Verification items for the finished model (mm, model axes). A direction names the side the tool comes from. Round coordinates to 2 decimals unless told otherwise and drop trailing zeros. Loops run counter-clockwise (first coordinate to the right, second up) from the corner with the lowest first, then second, coordinate; pieces in that order, holes last. Notation, with made-up numbers: M -38.5,53.25 L -0.5,53.25 A22 cw -0.5,65.25 Z; hole C -8.5,51 d3. An arc over 180 degrees is marked long. One line per item, written item: value.
from build123d import *

# Parameters (mm, degrees)
MODEL_R                 = 2
MODEL_R_2               = 1.5
MODEL_R_3               = 4.5
SALIENTE_EXTRUIR1_DEPTH = 3


with BuildPart() as part:
    # Model → Saliente-Extruir1 (new body)
    with BuildSketch(Plane.XY):
        with BuildLine():
            Line((53.427599038, 287.872856798), (56.220729127, 292.710700024))
            ThreePointArc((56.220729127, 292.710700024), (50.061313425, 295.08905988), (43.537923027, 296.109047676))
            Line((43.537923027, 296.109047676), (43.537923027, 290.522787498))
            Line((43.537923027, 290.522787498), (40.537923027, 290.522787498))
            Line((40.537923027, 290.522787498), (40.537923027, 296.109047676))
            ThreePointArc((40.537923027, 296.109047676), (34.014532629, 295.08905988), (27.855116927, 292.710700024))
            Line((27.855116927, 292.710700024), (30.648247016, 287.872856798))
            Line((30.648247016, 287.872856798), (28.050170805, 286.372856798))
            Line((28.050170805, 286.372856798), (25.257040716, 291.210700024))
            ThreePointArc((25.257040716, 291.210700024), (20.11761281, 287.065669482), (15.972582269, 281.926241576))
            Line((15.972582269, 281.926241576), (20.810425495, 279.133111488))
            Line((20.810425495, 279.133111488), (19.310425495, 276.535035276))
            Line((19.310425495, 276.535035276), (14.472582269, 279.328165365))
            ThreePointArc((14.472582269, 279.328165365), (12.094222412, 273.168749664), (11.074234616, 266.645359265))
            Line((11.074234616, 266.645359265), (16.660494794, 266.645359265))
            Line((16.660494794, 266.645359265), (16.660494794, 263.645359265))
            Line((16.660494794, 263.645359265), (11.074234616, 263.645359265))
            ThreePointArc((11.074234616, 263.645359265), (12.094222412, 257.121968867), (14.472582269, 250.962553166))
            Line((14.472582269, 250.962553166), (19.310425495, 253.755683255))
            Line((19.310425495, 253.755683255), (20.810425495, 251.157607043))
            Line((20.810425495, 251.157607043), (15.972582269, 248.364476954))
            ThreePointArc((15.972582269, 248.364476954), (20.11761281, 243.225049049), (25.257040716, 239.080018507))
            Line((25.257040716, 239.080018507), (28.050170805, 243.917861733))
            Line((28.050170805, 243.917861733), (30.648247016, 242.417861733))
            Line((30.648247016, 242.417861733), (27.855116927, 237.580018507))
            ThreePointArc((27.855116927, 237.580018507), (34.014532629, 235.20165865), (40.537923027, 234.181670855))
            Line((40.537923027, 234.181670855), (40.537923027, 239.767931032))
            Line((40.537923027, 239.767931032), (43.537923027, 239.767931032))
            Line((43.537923027, 239.767931032), (43.537923027, 234.181670855))
            ThreePointArc((43.537923027, 234.181670855), (50.061313425, 235.20165865), (56.220729127, 237.580018507))
            Line((56.220729127, 237.580018507), (53.427599038, 242.417861733))
            Line((53.427599038, 242.417861733), (56.025675249, 243.917861733))
            Line((56.025675249, 243.917861733), (58.818805338, 239.080018507))
            ThreePointArc((58.818805338, 239.080018507), (63.958233244, 243.225049049), (68.103263786, 248.364476954))
            Line((68.103263786, 248.364476954), (63.26542056, 251.157607043))
            Line((63.26542056, 251.157607043), (64.76542056, 253.755683255))
            Line((64.76542056, 253.755683255), (69.603263786, 250.962553166))
            ThreePointArc((69.603263786, 250.962553166), (71.981623642, 257.121968867), (73.001611438, 263.645359265))
            Line((73.001611438, 263.645359265), (67.41535126, 263.645359265))
            Line((67.41535126, 263.645359265), (67.41535126, 266.645359265))
            Line((67.41535126, 266.645359265), (73.001611438, 266.645359265))
            ThreePointArc((73.001611438, 266.645359265), (71.981623642, 273.168749664), (69.603263786, 279.328165365))
            Line((69.603263786, 279.328165365), (64.76542056, 276.535035276))
            Line((64.76542056, 276.535035276), (63.26542056, 279.133111488))
            Line((63.26542056, 279.133111488), (68.103263786, 281.926241576))
            ThreePointArc((68.103263786, 281.926241576), (63.958233244, 287.065669482), (58.818805338, 291.210700024))
            Line((58.818805338, 291.210700024), (56.025675249, 286.372856798))
            Line((56.025675249, 286.372856798), (53.427599038, 287.872856798))
        make_face()
        with Locations((42.037923027, 265.145359265)):
            Circle(MODEL_R, mode=Mode.SUBTRACT)
        with Locations((39.708551621, 273.838691702)):
            Circle(MODEL_R_2, mode=Mode.SUBTRACT)
        with Locations((44.367294433, 256.452026829)):
            Circle(MODEL_R_2, mode=Mode.SUBTRACT)
        with Locations((42.037923027, 281.644073382)):
            Circle(MODEL_R_3, mode=Mode.SUBTRACT)
        with Locations((27.749617473, 273.394716324)):
            Circle(MODEL_R_3, mode=Mode.SUBTRACT)
        with Locations((27.749617473, 256.896002207)):
            Circle(MODEL_R_3, mode=Mode.SUBTRACT)
        with Locations((42.037923027, 248.646645149)):
            Circle(MODEL_R_3, mode=Mode.SUBTRACT)
        with Locations((56.326228582, 256.896002207)):
            Circle(MODEL_R_3, mode=Mode.SUBTRACT)
        with Locations((56.326228582, 273.394716324)):
            Circle(MODEL_R_3, mode=Mode.SUBTRACT)
        with BuildLine():
            Line((47.354538273, 269.934589613), (45.664168077, 269.481656284))
            ThreePointArc((45.664168077, 269.481656284), (45.208763308, 269.132211915), (45.133837991, 268.563097631))
            Line((45.133837991, 268.563097631), (46.427933217, 263.733468499))
            ThreePointArc((46.427933217, 263.733468499), (46.777377587, 263.27806373), (47.34649187, 263.203138414))
            Line((47.34649187, 263.203138414), (49.036862066, 263.656071742))
            ThreePointArc((49.036862066, 263.656071742), (49.492266835, 264.005516112), (49.567192152, 264.574630396))
            Line((49.567192152, 264.574630396), (48.273096927, 269.404259527))
            ThreePointArc((48.273096927, 269.404259527), (47.923652557, 269.859664296), (47.354538273, 269.934589613))
        make_face(mode=Mode.SUBTRACT)
        with BuildLine():
            Line((35.038983988, 266.634646788), (36.729354184, 267.087580117))
            ThreePointArc((36.729354184, 267.087580117), (37.298468468, 267.0126548), (37.647912838, 266.557250031))
            Line((37.647912838, 266.557250031), (38.942008063, 261.7276209))
            ThreePointArc((38.942008063, 261.7276209), (38.867082746, 261.158506616), (38.411677977, 260.809062246))
            Line((38.411677977, 260.809062246), (36.721307781, 260.356128917))
            ThreePointArc((36.721307781, 260.356128917), (36.152193497, 260.431054234), (35.802749128, 260.886459003))
            Line((35.802749128, 260.886459003), (34.508653902, 265.716088135))
            ThreePointArc((34.508653902, 265.716088135), (34.583579219, 266.285202419), (35.038983988, 266.634646788))
        make_face(mode=Mode.SUBTRACT)
    extrude(amount=SALIENTE_EXTRUIR1_DEPTH)


solid = part.part
(1) Tool access check on faces 3 (the face through (43.538, 293, 1)), 4 (the face through (37.578, 260.586, 1.479)), 5 (the face through (40.538, 237, 1)), 6 (the face through (50.151, 295.065, 1.479)). Record the directions out of +Z, -Z, +X, -X, +Y, -Y that give a thin tool (end or side, any length) a straight path to the whole face; none if there is none.
Completed:
face 3: +Z, -Z, +Y
face 4: +Z, -Z
face 5: +Z, -Z, -Y
face 6: +Z, -Z, +X, +Y
(2) Thickness scan on L1, parallel to X at y = 289.5, z = 0.55; L2, parallel to Y at x = 30, z = 1.95; L3, parallel to X at y = 278.5, z = 0.7. Record the ranges inside material, lowest first. Write a range as from..to.
Completed:
L1: x = 22.86..26.24, 29.71..54.37, 57.83..61.22
L2: y = 236.58..241.3, 242.79..253, 260.79..269.5, 277.29..287.5, 289..293.71
L3: x = 14.06..15.91, 20.44..38.82, 45.26..63.63, 68.17..70.01
(3) Sectioned sample at C-C on z = 2.2. Count the separate pieces of the cut face and the enclosed holes in it, and give its area (3 significant figures).
Completed:
separate pieces: 1
enclosed holes: 11
area: 2,370 mm^2
(4) Depth check by flat-ended pin: pin 1 Ø7 at (x, y) = (27.75, 256.9) entering from -Z; pin 2 Ø0.9 at (y, z) = (238.5, 1.5) entering from -X; pin 3 Ø0.9 at (x, z) = (14.5, 1) entering from +Y; pin 4 Ø1 at (x, z) = (39, 1) entering from -Y. Enter the tip coordinate at first touch or a pass-through.
Completed:
pin 1: passes through
pin 2: stops at x = 28.13
pin 3: stops at y = 279.33
pin 4: stops at y = 234.25
(5) Mould release check, pull along X, two halves, no side actions. Record for faces 1 (the face through (42, 239.768, 1)), 2 (the face through (67.415, 265, 1)): +X half, -X half, draft (parallel to the pull), parting line (faces both ways), or undercut.
Completed:
face 1: undercut
face 2: +X half
(6) Sectioned sample at D-D on x = 22.5. Enter the section's corners in (y, z), and give its area (3 significant figures).
Completed:
outline: M 241.08,0 L 289.21,0 L 289.21,3 L 241.08,3 Z
area: 144 mm^2
(7) Sectioned sample at B-B on y = 241.5. Enter the section's corners in (x, z), and give its area (3 significant figures).
Completed:
outline: M 21.99,0 L 26.65,0 L 26.65,3 L 21.99,3 Z; M 30.12,0 L 53.96,0 L 53.96,3 L 30.12,3 Z; M 57.42,0 L 62.09,0 L 62.09,3 L 57.42,3 Z
area: 99.5 mm^2
(8) Sectioned sample at A-A on x = 60. Enter the section's corners in (y, z), and give its area (3 significant figures).
Completed:
outline: M 239.88,0 L 254.3,0 L 254.3,3 L 239.88,3 Z; M 259.49,0 L 270.8,0 L 270.8,3 L 259.49,3 Z; M 275.99,0 L 290.41,0 L 290.41,3 L 275.99,3 Z
area: 120 mm^2
